Autodesk Inventor part; units mm, degrees
ref_plane "fix_end_r_XY" through (0, 17, 0) normal (0, 0, 1) x (1, 0, 0)
ref_plane "fix_end_r_YZ" through (0, 17, 0) normal (1, 0, 0) x (0, 1, 0)
ref_plane "fix_end_r_ZX" through (0, 17, 0) normal (0, 1, 0) x (0, 0, 1)
sketch "Sketch_10" plane through (0, 0, 0) normal (0, 0, 1) x (1, 0, 0)
  arc A0 (-16.7417, 19.952) -> (7.4171, 1.7034) centre (0, 17) ccw
  line L0 (7.4171, 1.7034) -> (58.0834, 26.2707)
  arc A1 (58.0834, 26.2707) -> (60, 29.33) centre (56.6, 29.33) ccw
  line L1 (60, 29.33) -> (60, 34)
  line L2 (60, 34) -> (0, 34)
  arc A2 (0, 34) -> (-12.0208, 29.0208) centre (0, 17) ccw
  line L3 (-12.0208, 29.0208) -> (-5.3033, 22.3033)
  arc A3 (-5.3033, 22.3033) -> (-7.3861, 18.3024) centre (0, 17) ccw
  line L4 (-7.3861, 18.3024) -> (-16.7417, 19.952)
  circle A4 centre (0, 17) radius 4.25
extrude "Extrusion1" add sketch "Sketch_10" along normal blind 20
sketch "Sketch_1" plane through (0, 0, 0) normal (1, 0, 0) x (0, 1, 0)
  line L0 (39, 25) -> (-5, 25)
  line L1 (-5, 25) -> (-5, -5)
  line L2 (-5, -5) -> (39, -5)
  line L3 (39, -5) -> (39, 25)
  line L4 (34, 20) -> (32, 20)
  line L5 (32, 20) -> (32, 3)
  arc A0 (31, 2) -> (32, 3) centre (31, 3) ccw
  line L6 (31, 2) -> (0, 2)
  line L7 (0, 2) -> (0, 0)
  line L8 (0, 0) -> (32, 0)
  arc A1 (32, 0) -> (34, 2) centre (32, 2) ccw
  line L9 (34, 2) -> (34, 20)
extrude "Extrusion2" cut sketch "Sketch_1" along normal mid plane 188
sketch "Sketch_3" plane through (0, 0, 0) normal (0, 1, 0) x (-1, 0, 0)
  line L0 (22, 25) -> (-65, 25)
  line L1 (-65, 25) -> (-65, -5)
  line L2 (-65, -5) -> (22, -5)
  line L3 (22, -5) -> (22, 25)
  line L4 (17, 2) -> (-20, 2)
  line L5 (-20, 2) -> (-20, 15)
  arc A0 (-20, 15) -> (-25, 20) centre (-25, 15) ccw
  line L6 (-25, 20) -> (-55, 20)
  arc A1 (-55, 20) -> (-60, 15) centre (-55, 15) ccw
  line L7 (-60, 15) -> (-60, 0)
  line L8 (-60, 0) -> (17, 0)
  line L9 (17, 0) -> (17, 2)
extrude "Extrusion3" cut sketch "Sketch_3" along normal blind 34
sketch "Sketch_2" plane through (0, 34, 0) normal (0, 1, 0) x (1, 0, 0)
  circle A0 centre (28, -10) radius 3.5
extrude "Extrusion4" cut sketch "Sketch_2" along normal mid plane 4
sketch "Sketch_4" plane through (0, 34, 0) normal (0, 1, 0) x (1, 0, 0)
  circle A0 centre (52, -10) radius 3.5
extrude "Extrusion5" cut sketch "Sketch_4" along normal mid plane 4
sketch "Sketch_7" plane through (0, 0, 0) normal (0, 0, 1) x (1, 0, 0)
  circle A0 centre (15, 34) radius 2.5
extrude "Extrusion6" cut sketch "Sketch_7" along normal blind 20
ref_plane "fix_end_r_XY" through (0, 17, 0) normal (0, 0, 1) x (1, 0, 0)
ref_plane "fix_end_r_YZ" through (0, 17, 0) normal (1, 0, 0) x (0, 1, 0)
ref_plane "fix_end_r_ZX" through (0, 17, 0) normal (0, 1, 0) x (0, 0, 1)
ref_plane "free_end_r_XY" through (0, 17, 2) normal (0, 0, 1) x (1, 0, 0)
ref_plane "free_end_r_YZ" through (0, 17, 2) normal (1, 0, 0) x (0, 1, 0)
ref_plane "free_end_r_ZX" through (0, 17, 2) normal (0, 1, 0) x (0, 0, 1)
ref_plane "r_XY" through (0, 17, 27.8) normal (0, 0, 1) x (1, 0, 0)
ref_plane "r_YZ" through (0, 17, 27.8) normal (1, 0, 0) x (0, 1, 0)
ref_plane "r_ZX" through (0, 17, 27.8) normal (0, 1, 0) x (0, 0, 1)
properties part number "MHPUS306-Ab_free_right"
For this review, take the finished solid that the model builds, in its own axes (mm). A direction names the side the tool comes from. Coordinates: 2 decimals unless noted, no trailing zeros. Write each loop counter-clockwise with the first axis right and the second up, starting at its lowest first coordinate (ties: lowest second). Pieces come first, ordered by that corner, then holes.
(1) Add section D-D on x = -2.5. Give the boundary of the cut face in (y, z).
(2) Tool access review of faces 5 (the face through (-6.67, 20.43, 0.99)), 6 (the face through (40, 32, 12)), 7 (the face through (-9, 26, 1)): name each direction out of +Z, -Z, +X, -X, +Y, -Y from which nothing blocks a thin tool from reaching the whole face with its end or side.
(3) Add section C-C on x = 54. Give the boundary of the cut face in (y, z), then the cut area to 3 significant figures.
(4) Wall thickness on probe 1 along X at (y, z) = (33.3, 10); probe 2 along Z at (x, y) = (16, 11); probe 3 along Y at (x, z) = (33.5, 7): over which ranges is each line inside the solid? List them lowest first.
(5) Add section B-B on y = 17. Give the boundary of the cut face in (x, z).
(6) The part is to be moulded in two halves that separate along Y. For faces 1 (the face through (59.495, 27.548, 0.986)), 2 (the face through (22, 33, 19)), 3 (the face through (15.1, 31.5, 1)), 4 (the face through (-11.998, 19.116, 0.986)), say which applies: +Y half, -Y half, draft (parallel to the pull), parting line (faces both ways), or undercut.
(7) Add section A-A on z = 10. Give the boundary of the cut face in (x, y).
(8) For pin 1 Ø12 at (y, z) = (28, 13.5) entering from +X; pin 2 Ø5.5 at (x, z) = (52, 10) entering from +Y; pin 3 Ø8.5 at (x, z) = (35.5, 9) entering from -Y; pin 4 Ø17 at (x, y) = (10.5, 12.5) entering from +Z, all flat-tipped, find the tip position at first contact; note any pin that passes through.
Answer sheet:
1. outline: (0.18, 0) - (13.56, 0) - (13.56, 2) - (0.18, 2) - close; (20.44, 0) - (32, 0) arc R2 ccw to (33.82, 1.16) - (33.82, 2) - (20.44, 2) - close
2. face 5: +Z, -Z
2. face 6: +Z, +X, -X, -Y
2. face 7: +Z, -Z, -X
3. outline: (24.29, 0) - (32, 0) arc R2 ccw to (34, 2) - (34, 7.13) - (32, 7.13) - (32, 3) arc R1 cw to (31, 2) - (24.29, 2) - close; (32, 12.87) - (34, 12.87) - (34, 20) - (32, 20) - close
3. area: 43.3 mm2
4. probe 1: x = 20 to 24.5, 31.5 to 48.5, 55.5 to 60
4. probe 2: z = 0 to 2
4. probe 3: y = 32 to 34
5. outline: (-17, 0) - (-4.25, 0) - (-4.25, 2) - (-17, 2) - close; (4.25, 0) - (38.96, 0) - (38.96, 2) - (4.25, 2) - close
6. face 1: -Y half
6. face 2: draft
6. face 3: +Y half
6. face 4: undercut
7. outline: (20, 32) - (24.5, 32) - (24.5, 34) - (20, 34) - close; (31.5, 32) - (48.5, 32) - (48.5, 34) - (31.5, 34) - close; (55.5, 32) - (60, 32) - (60, 34) - (55.5, 34) - close
8. pin 1: stops at x = 60
8. pin 2: passes through
8. pin 3: stops at y = 32
8. pin 4: stops at z = 2
